```python
from build123d import *

# Parameters (mm, degrees)
SKETCH_R      = 26
SKETCH_R_2    = 10.5
PAD_DEPTH     = 2
SKETCH001_R   = 25
SKETCH001_R_2 = 10.5
PAD001_DEPTH  = 8.5
SKETCH004_R   = 12.5
POCKET_DEPTH  = 2


with BuildPart() as part:
    # Sketch → Pad (new body)
    with BuildSketch(Plane.XY):
        Circle(SKETCH_R)
        Circle(SKETCH_R_2, mode=Mode.SUBTRACT)
    extrude(amount=PAD_DEPTH)

    # Sketch001 → Pad001 (join)
    with BuildSketch(Plane.XY):
        Circle(SKETCH001_R)
        Circle(SKETCH001_R_2, mode=Mode.SUBTRACT)
    extrude(amount=PAD001_DEPTH)

    # Sketch002 → SubtractiveLoft section 0
    with BuildSketch(Plane.XY):
        Polygon((1, 23), (-1, 23), (-1, 1), (-23, 1), (-23, -1), (-1, -1), (-1, -23), (1, -23), (1, -1), (23, -1), (23, 1), (1, 1), align=None)
    # Sketch003 → SubtractiveLoft section 1
    with BuildSketch(Plane.XY.offset(12)):
        Polygon((1, 13), (-1, 13), (-1, 1), (-13, 1), (-13, -1), (-1, -1), (-1, -13), (1, -13), (1, -1), (13, -1), (13, 1), (1, 1), align=None)
    loft(mode=Mode.SUBTRACT)

    # Sketch004 → Pocket (cut)
    with BuildSketch(Plane.XY):
        Circle(SKETCH004_R)
    extrude(amount=POCKET_DEPTH, mode=Mode.SUBTRACT)


solid = part.part
```
Design review of the part built by this model. Coordinates are the model's own, in mm. A direction names the side the tool comes from. Coordinates: 2 decimals unless noted, no trailing zeros. Order: outer loops, then holes, each group sorted by start corner. A loop starts at its lowest first (then second) coordinate and runs counter-clockwise, first axis right, second up. Notation, with made-up numbers: (-9, 22) -> (30, 22) arc R20 ccw to (30, 45) -> close; hole circle Ø3 at (56.25, 8.5). An arc over 180 degrees is marked (long way). One line per item, written item: value. Start each with the question number.
Q1. For probe 1 along X at (y, z) = (6, 5.5); probe 2 along X at (y, z) = (-7, 4.75); probe 3 along Y at (x, z) = (14, 1.5), list the stretches that pass through material, from the lowest coordinate up.
Q2. Insertion check: pin 1 Ø3.5 at (x, y) = (-8.5, 4.5) entering from -Z; pin 2 Ø1.5 at (y, z) = (-11.5, 3) entering from +X; pin 3 Ø5 at (y, z) = (5, 2.5) entering from +X. Each pin has a flat end and moves straight along its axis. Give the tip position at first contact, or say it passes through.
Q3. Take a section at D-D, the plane x = 6.5. State the section outline as (y, z) points, then the cut area to 3 significant figures.
Q4. Take a section at C-C, the plane x = -6. State the section outline as (y, z) points, then the cut area to 3 significant figures.
Q5. Tool access review of faces 4 (the flat face through (19.41, -0.01, 4.31)), 5 (the cylindrical face through (-7.35, 7.5, 5.2)), 6 (the flat face through (11.2, 6.1, 0)): name each direction out of +Z, -Z, +X, -X, +Y, -Y from which nothing blocks a thin tool from reaching the whole face with its end or side.
Q6. Mouldability with a two-part tool opening along X and no side actions: class faces 1 (the flat face through (-0.01, -19.41, 4.31)), 2 (the cylindrical face through (-20.633, -15.821, 0.986)), 3 (the flat face through (-14, 21, 2)) as pulls with the +X half, pulls with the -X half, needs draft (parallel to the pull), parting line crosses it, or undercut.
Q7. Take a section at A-A, the plane y = 0. State the section outline as (x, z) points.
Values follow:
1. probe 1: x = -24.27 to -8.62, 8.62 to 24.27
1. probe 2: x = -24 to -7.83, 7.83 to 24
1. probe 3: y = -21.91 to -1, 1 to 21.91
2. pin 1: stops at z = 2
2. pin 2: stops at x = 22.57
2. pin 3: stops at x = 25.87
3. outline: (-25.17, 0) -> (-10.68, 0) -> (-10.68, 2) -> (-8.25, 2) -> (-8.25, 8.5) -> (-24.14, 8.5) -> (-24.14, 2) -> (-25.17, 2) -> close; (8.25, 2) -> (10.68, 2) -> (10.68, 0) -> (25.17, 0) -> (25.17, 2) -> (24.14, 2) -> (24.14, 8.5) -> (8.25, 8.5) -> close
3. area: 265 mm2
4. outline: (-25.3, 0) -> (-10.97, 0) -> (-10.97, 2) -> (-8.62, 2) -> (-8.62, 8.5) -> (-24.27, 8.5) -> (-24.27, 2) -> (-25.3, 2) -> close; (8.62, 2) -> (10.97, 2) -> (10.97, 0) -> (25.3, 0) -> (25.3, 2) -> (24.27, 2) -> (24.27, 8.5) -> (8.62, 8.5) -> close
4. area: 261 mm2
5. face 4: -Z
5. face 5: +Z, -Z
5. face 6: -Z, +X, -X, +Y, -Y
6. face 1: undercut
6. face 2: parting line crosses it
6. face 3: needs draft
7. outline: (-26, 0) -> (-23, 0) -> (-15.92, 8.5) -> (-25, 8.5) -> (-25, 2) -> (-26, 2) -> close; (15.92, 8.5) -> (23, 0) -> (26, 0) -> (26, 2) -> (25, 2) -> (25, 8.5) -> close
